Work out the finished part from the listing and answer in its coordinate system (mm). Face numbers are marked on the shaded views. A direction names the side the tool comes from. Round coordinates to 2 decimals unless told otherwise and drop trailing zeros. Order: outer loops, then holes, each group sorted by start corner. A loop starts at its lowest first (then second) coordinate and runs counter-clockwise, first axis right, second up. Notation, with made-up numbers: (23, -3) - (82, -3) arc R29 ccw to (82, 31) - close; hole circle Ø8 at (47.5, 35). An arc over 180 degrees is marked (long way). Answer in a Markdown table with one row per item.
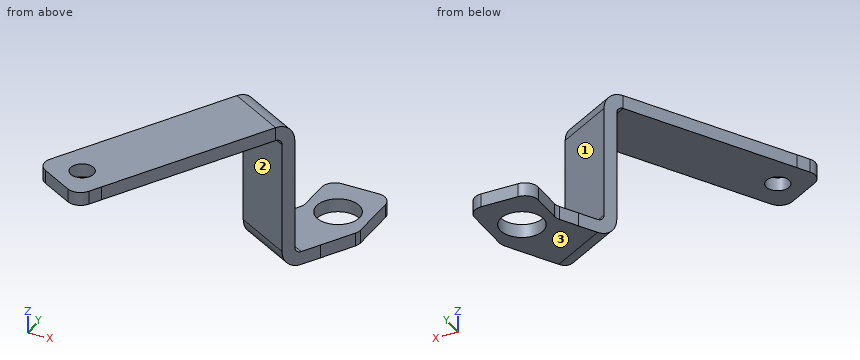
from build123d import *

# Parameters (mm, degrees)
BASE_FLANGE1_DEPTH   = 3.175
EDGE_FLANGE1_DEPTH   = 15
EDGE_FLANGE2_DEPTH   = 15
SKETCH15_R           = 5.08
BOSS_EXTRUDE1_DEPTH  = 3.175
M5_CLEARANCE_HOLE1_D = 5.5
FILLET1_R            = 3.175


# Sheet-metal steps are written as plain solids
with BuildPart() as part:
    # Sketch2 → Base-Flange1 (new body)
    with BuildSketch(Plane.XY):
        Polygon((-136.862074611, 27.127820722), (-140.037074611, 21.628559408), (-153.027455668, 29.128559408), (-149.852455668, 34.627820722), (-128.262455668, 72.022797657), (-115.272074611, 64.522797657), align=None)
    extrude(amount=BASE_FLANGE1_DEPTH)

    # Edge-Flange1 section (across the edge) → Edge-Flange1 (add)
    with BuildSketch(Plane(origin=(-127.468705668, 73.397612986, 0), x_dir=(-0.49999999999999706, -0.8660254037844404, -3.491481338843133e-15), z_dir=(0.8660254037844404, -0.49999999999999706, 0))):
        with BuildLine():
            Line((-3.175, 1.5875), (-3.175, 27.899995))
            Line((-3.175, 27.899995), (0, 27.899995))
            Line((0, 27.899995), (0, 1.5875))
            ThreePointArc((0, 1.5875), (0.464967985, 0.464967985), (1.5875, 0))
            Line((1.5875, 0), (1.5875, -3.175))
            ThreePointArc((1.5875, -3.175), (-1.780096045, -1.780096045), (-3.175, 1.5875))
        make_face()
    extrude(amount=EDGE_FLANGE1_DEPTH)

    # Edge-Flange2 section (across the edge) → Edge-Flange2 (add)
    with BuildSketch(Plane(origin=(-112.890824611, 68.647243643, -29.487495), x_dir=(0, 0, 1), z_dir=(-0.8660254037844405, 0.4999999999999967, 0))):
        with BuildLine():
            Line((-3.175, 1.5875), (-3.175, 6.35))
            Line((-3.175, 6.35), (0, 6.35))
            Line((0, 6.35), (0, 1.5875))
            ThreePointArc((0, 1.5875), (0.464967985, 0.464967985), (1.5875, 0))
            Line((1.5875, 0), (1.5875, -3.175))
            ThreePointArc((1.5875, -3.175), (-1.780096045, -1.780096045), (-3.175, 1.5875))
        make_face()
    extrude(amount=EDGE_FLANGE2_DEPTH)

    # Sketch15 → Boss-Extrude1 (add)
    with BuildSketch(Plane(origin=(0, 0, -32.662495), x_dir=(-1, 0, 0), z_dir=(0, 0, -1))):
        Polygon((122.706205668, 81.646504957), (109.715824611, 74.146504957), (104.953324611, 82.395396928), (104.953324611, 97.635396928), (119.953324611, 97.635396928), (119.953324611, 86.414634815), align=None)
        with Locations((112.453324611, 87.475396928)):
            Circle(SKETCH15_R, mode=Mode.SUBTRACT)
    extrude(amount=-BOSS_EXTRUDE1_DEPTH)

    # M5 Clearance Hole1 (through all)
    with Locations(Plane.XY.offset(3.175)):
        with Locations((-143.35726514, 30.877820722)):
            Hole(M5_CLEARANCE_HOLE1_D / 2)

    # Fillet1
    fillet1_edges = [part.edges().sort_by_distance(p)[0] for p in [
        (-140.037074611, 21.628559408, 1.5875),
        (-153.027455668, 29.128559408, 1.5875),
        (-119.953324611, 86.414634815, -31.074995),
        (-104.953324611, 82.395396928, -31.074995),
        (-104.953324611, 97.635396928, -31.074995),
        (-119.953324611, 97.635396928, -31.074995),
    ]]
    fillet(fillet1_edges, radius=FILLET1_R)


solid = part.part
1) Find the intervals of material crossed by probe 1 along Z at (x, y) = (-142.5, 45.5) (3 decimals); probe 2 along Z at (x, y) = (-114.5, 72); probe 3 along Y at (x, z) = (-117.5, -25), in increasing order. Write a range as from..to.
Filled in:
| item | result |
|---|---|
| probe 1 | z = 0..3.175 |
| probe 2 | z = -32.66..-29.49 |
| probe 3 | y = 67.64..71.31 |
2) Which of the six approach directions +Z, -Z, +X, -X, +Y, -Y give full straight-line access (tool end or side, diameter ignored) to the marked faces 1, 2 and 3?
Filled in:
| item | result |
|---|---|
| face 1 | +Z, +X, +Y |
| face 2 | -Z, -X, -Y |
| face 3 | -Z, +X, -X, +Y, -Y |
3) Find section B-B, the plane y = 41.5. Give the vertices of the cut face in (x, z) (3 decimals).
Filled in:
| item | result |
|---|---|
| outline | (-145.885, 0) - (-128.564, 0) - (-128.564, 3.175) - (-145.885, 3.175) - close |
4) Each of these flat-tipped pins is pushed along its axis until it touches: pin 1 (8 mm diameter, centred on x = -126, y = 50.5, fed in from -Z); pin 2 (1.5 mm diameter, centred on x = -113.5, z = -16, fed in from -Y); pin 3 (8 mm diameter, centred on y = 44, z = -1.5, fed in from +X); pin 4 (9 mm diameter, centred on x = -112.45, y = 87.48, fed in from -Z). Where does it stop, or does it pass through?
Filled in:
| item | result |
|---|---|
| pin 1 | stops at z = 0 |
| pin 2 | stops at y = 66.29 |
| pin 3 | stops at x = -124.98 |
| pin 4 | passes through |
5) Find section A-A, the plane z = -24.5. Give the vertices of the cut face in (x, y), then the cut area to 3 significant figures.
Filled in:
| item | result |
|---|---|
| outline | (-127.47, 73.4) - (-114.48, 65.9) - (-112.89, 68.65) - (-125.88, 76.15) - close |
| area | 47.6 mm^2 |
